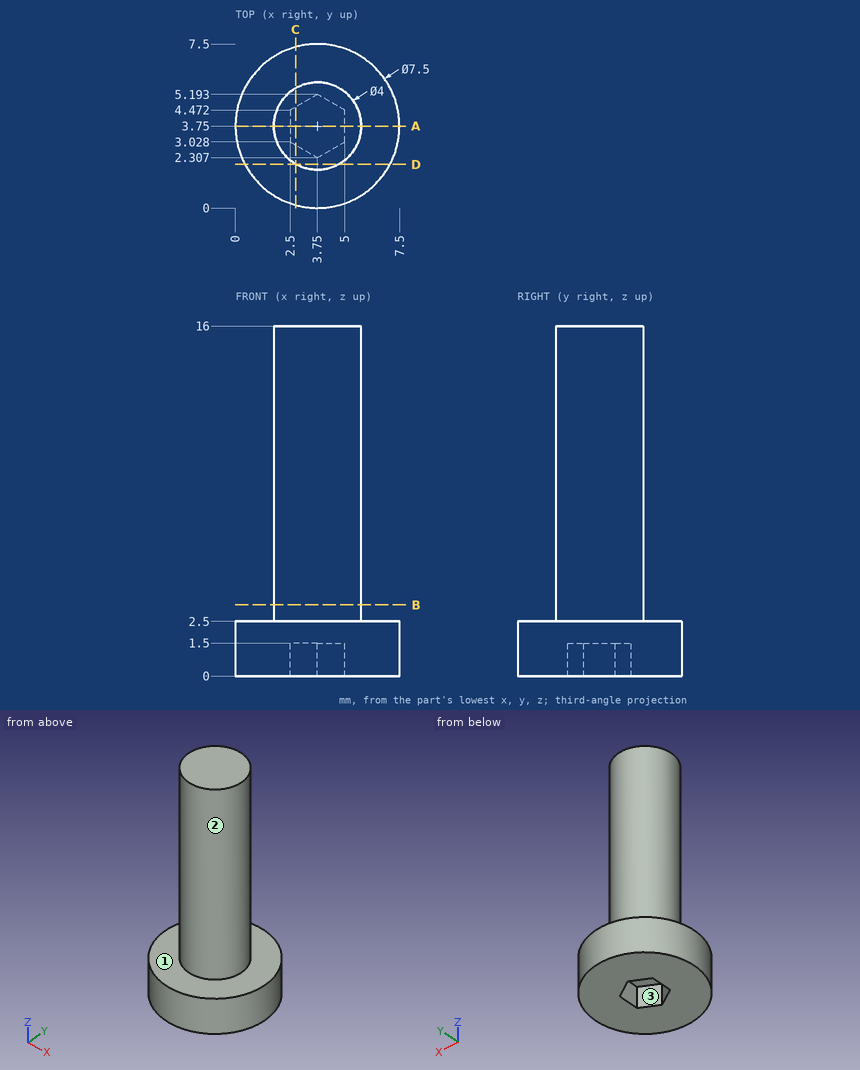
Print and shaded views of the part. All mm, measured from the part's lowest x, y and z. Round coordinates to 2 decimals unless told otherwise and drop trailing zeros. Write each loop counter-clockwise with the first axis right and the second up, starting at its lowest first coordinate (ties: lowest second). Pieces come first, ordered by that corner, then holes.
(1) Drop flat-ended pins along their axis: P1, Ø1, axis at x = 1, z = 5.5, coming from the +Y side; P2, Ø2, axis at x = 4.5, z = 5.5, coming from the -Y side; P3, Ø4, axis at y = 3, z = 12, coming from the +X side. Give the stop position or say it passes through.
(2) Slice it at C-C, the plane x = 2.75. Write the cut outline in (y, z).
(3) Slice it at D-D, the plane y = 2. Write the cut outline in (x, z).
(4) Mould opens along Y. For the marked faces 1, 2 and 3 say: pulls with the +Y half, pulls with the -Y half, needs draft (parallel to the pull), parting line crosses it, or undercut.
(5) Slice it at B-B, the plane z = 3.25. Write the cut outline in (x, y), and give its area (3 significant figures).
(6) Slice it at A-A, the plane y = 3.75. Write the cut outline in (x, z).
(7) Probe line 1 along Z through (x, y) = (5.5, 6.75); line 2 along Z through (x, y) = (3, 4.25); line 3 along Y through (x, z) = (3.75, 3.5). List the from-to ranges inside material, lowest first.
From the geometry:
1. P1: passes through
1. P2: stops at y = 1.75
1. P3: stops at x = 5.75
2. outline: (0.14, 0) - (2.88, 0) - (2.88, 1.5) - (4.62, 1.5) - (4.62, 0) - (7.36, 0) - (7.36, 2.5) - (5.48, 2.5) - (5.48, 16) - (2.02, 16) - (2.02, 2.5) - (0.14, 2.5) - close
3. outline: (0.43, 0) - (7.07, 0) - (7.07, 2.5) - (4.72, 2.5) - (4.72, 16) - (2.78, 16) - (2.78, 2.5) - (0.43, 2.5) - close
4. face 1: needs draft
4. face 2: parting line crosses it
4. face 3: undercut
5. outline: circle Ø4 at (3.75, 3.75)
5. area: 12.6 mm2
6. outline: (0, 0) - (2.5, 0) - (2.5, 1.5) - (5, 1.5) - (5, 0) - (7.5, 0) - (7.5, 2.5) - (5.75, 2.5) - (5.75, 16) - (1.75, 16) - (1.75, 2.5) - (0, 2.5) - close
7. line 1: z = 0 to 2.5
7. line 2: z = 1.5 to 16
7. line 3: y = 1.75 to 5.75
